Read the model definition and answer for the solid it produces. Units are mm, in the model's axes. Round coordinates to 2 decimals unless told otherwise and drop trailing zeros. Order: outer loops, then holes, each group sorted by start corner. A loop starts at its lowest first (then second) coordinate and runs counter-clockwise, first axis right, second up. Notation, with made-up numbers: (78, 55) -> (135, 55) arc R7 ccw to (135, 62) -> close; hole circle Ø2 at (3.5, 57). An arc over 180 degrees is marked (long way). One line per item, written item: value. Start each with the question number.
1. Section A-A (y = -1.05) is taken. State how many separate pieces and enclosed holes the cut face has, then the cut area to 3 significant figures.
2. Consider line 1 (X direction, y = -4.7, z = -52.5); line 2 (X direction, y = -3, z = -73.5); line 3 (Z direction, x = -41, y = -4.2). Determine where each line is inside the solid, lowest interval first.
3. A flat-ended cylindrical pin translates along its axis: pin 1 Ø2.5 at (x, z) = (71.7, -29.7) entering from -Y. Find the tip coordinate at first contact, or state that the pin passes through.
4. Section C-C (x = 43) is taken. Give the vertices of the cut face in (y, z).
5. Section B-B (z = -52) is taken. Give the vertices of the cut face in (x, y), then the cut area to 3 significant figures.
Autodesk Inventor part; units mm, degrees
ref_plane "YZ Plane" through (0, 0, 0) normal (1, 0, 0) x (0, 1, 0)
ref_plane "XZ Plane" through (0, 0, 0) normal (0, 1, 0) x (-1, 0, 0)
ref_plane "XY Plane" through (0, 0, 0) normal (0, 0, 1) x (1, 0, 0)
ref_plane "Work Plane13" through (0, 0, 0) normal (0, -1, 0) x (1, 0, 0)
sketch "Sketch13" plane through (0, 0, 0) normal (0, -1, 0) x (1, 0, 0)
  circle A0 centre (-71.6992, -29.6988) radius 0.75
  circle A1 centre (29.6988, -71.6992) radius 0.75
  circle A2 centre (71.6992, 29.6988) radius 0.75
  circle A3 centre (29.6988, 71.6992) radius 0.75
  circle A4 centre (-29.6988, 71.6992) radius 0.75
  circle A5 centre (71.6992, -29.6988) radius 0.75
  circle A6 centre (-29.6988, -71.6992) radius 0.75
  circle A7 centre (-71.6992, 29.6988) radius 0.75
  line L0 (-82.6875, -34.2503) -> (-34.2503, -82.6875)
  line L1 (-34.2503, -82.6875) -> (34.2503, -82.6875)
  line L2 (34.2503, -82.6875) -> (82.6875, -34.2503)
  line L3 (82.6875, -34.2503) -> (82.6875, 34.2503)
  line L4 (82.6875, 34.2503) -> (34.2503, 82.6875)
  line L5 (34.2503, 82.6875) -> (-34.2503, 82.6875)
  line L6 (-34.2503, 82.6875) -> (-82.6875, 34.2503)
  line L7 (-82.6875, 34.2503) -> (-82.6875, -34.2503)
  arc A8 (-33.3536, 70.0737) -> (-25.965, 73.1342) centre (-29.6988, 71.6992) ccw
  arc A9 (25.965, 73.1342) -> (-25.965, 73.1342) centre (0, 0) ccw
  arc A10 (25.965, 73.1342) -> (33.3536, 70.0737) centre (29.6988, 71.6992) ccw
  arc A11 (70.0737, 33.3536) -> (33.3536, 70.0737) centre (0, 0) ccw
  arc A12 (70.0737, 33.3536) -> (73.1342, 25.965) centre (71.6992, 29.6988) ccw
  arc A13 (73.1342, -25.965) -> (73.1342, 25.965) centre (0, 0) ccw
  arc A14 (73.1342, -25.965) -> (70.0737, -33.3536) centre (71.6992, -29.6988) ccw
  arc A15 (33.3536, -70.0737) -> (70.0737, -33.3536) centre (0, 0) ccw
  arc A16 (33.3536, -70.0737) -> (25.965, -73.1342) centre (29.6988, -71.6992) ccw
  arc A17 (-25.965, -73.1342) -> (25.965, -73.1342) centre (0, 0) ccw
  arc A18 (-25.965, -73.1342) -> (-33.3536, -70.0737) centre (-29.6988, -71.6992) ccw
  arc A19 (-70.0737, -33.3536) -> (-33.3536, -70.0737) centre (0, 0) ccw
  arc A20 (-70.0737, -33.3536) -> (-73.1342, -25.965) centre (-71.6992, -29.6988) ccw
  arc A21 (-73.1342, 25.965) -> (-73.1342, -25.965) centre (0, 0) ccw
  arc A22 (-73.1342, 25.965) -> (-70.0737, 33.3536) centre (-71.6992, 29.6988) ccw
  arc A23 (-33.3536, 70.0737) -> (-70.0737, 33.3536) centre (0, 0) ccw
extrude "Extrusion11" add sketch "Sketch13" along normal blind 5 contours L7 L6 L5 L4 L3 L2 L1 L0 | A8 A9 A10 A11 A12 A13 A14 A15 A16 A17 A18 A19 A20 A21 A22 A23
chamfer "Chamfer2" distance 1 angle 45 8 edges at (-72.4492, -5, -29.6988) (-30.4488, -5, -71.6992) (28.9488, -5, -71.6992) (70.9492, -5, -29.6988) (70.9492, -5, 29.6988) (28.9488, -5, 71.6992) (-30.4488, -5, 71.6992) (-72.4492, -5, 29.6988)
properties part number "meteostanica radiation shield spodny kryt"
Answer:
1. separate pieces: 1
1. enclosed holes: 8
1. area: 22,600 mm^2
2. line 1: -64.44 to 64.44
2. line 2: -43.44 to 43.44
2. line 3: -75.94 to 75.94
3. pin 1: y = -4.5
4. outline: (-5, -73.94) -> (0, -73.94) -> (0, 73.94) -> (-5, 73.94) -> close
5. outline: (-64.94, -5) -> (64.94, -5) -> (64.94, 0) -> (-64.94, 0) -> close
5. area: 649 mm^2
